The figure shows three views and two pictorial views of one solid part (mm, origin at its lowest corner). Answer the questions. Coordinates: 2 decimals unless noted, no trailing zeros. Loops run counter-clockwise (first coordinate to the right, second up) from the corner with the lowest first, then second, coordinate; pieces in that order, holes last. Notation, with made-up numbers: (-8, 8) -> (5, 8) arc R24 ccw to (5, 23) -> close; hole circle Ø4 at (27.25, 27.25). An arc over 180 degrees is marked (long way). Answer in a Markdown table with one row per item.
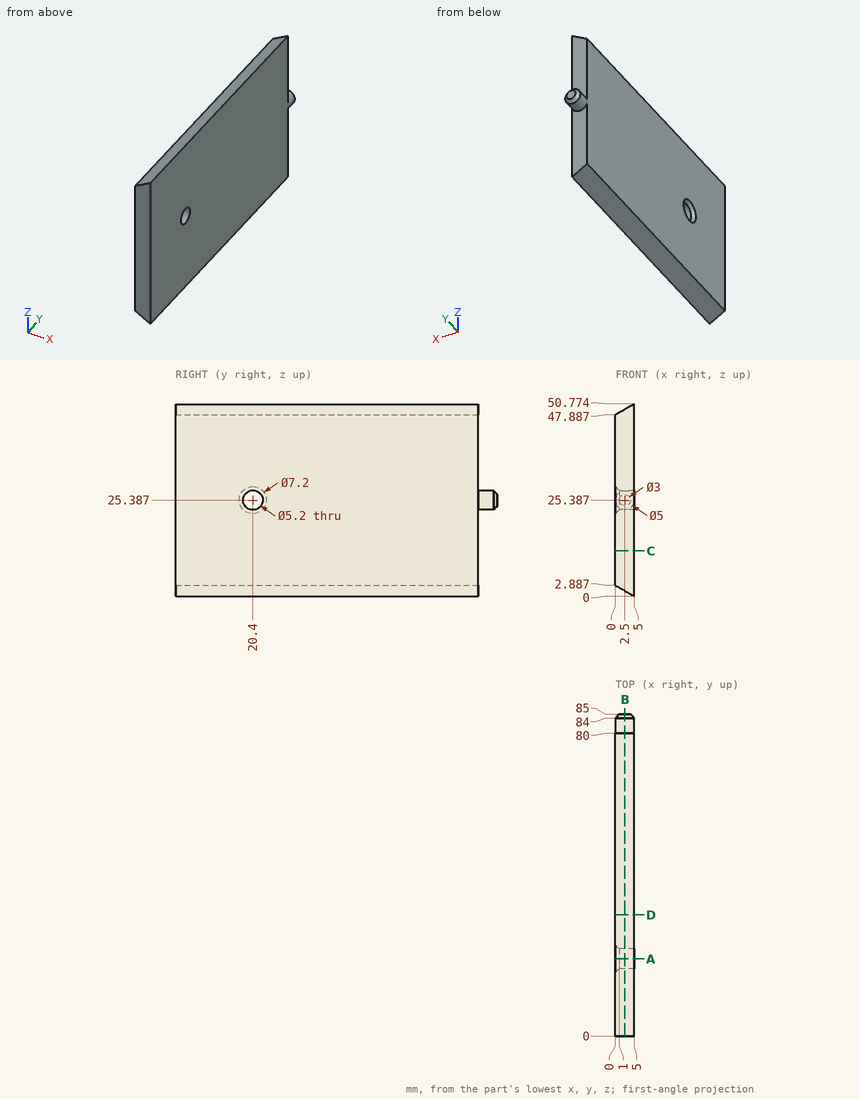
Item 1: A cutting plane is placed at B-B, the plane x = 2.5. Determine the outline of the cut face in (y, z).
Findings below:
| item | result |
|---|---|
| outline | (0, 1.44) -> (80, 1.44) -> (80, 22.89) -> (84, 22.89) -> (85, 23.89) -> (85, 26.89) -> (84, 27.89) -> (80, 27.89) -> (80, 49.33) -> (0, 49.33) -> close; hole circle Ø5.2 at (20.4, 25.39) |
Item 2: A cutting plane is placed at D-D, the plane y = 32. Determine the outline of the cut face in (x, z).
Findings below:
| item | result |
|---|---|
| outline | (0, 2.89) -> (5, 0) -> (5, 50.77) -> (0, 47.89) -> close |
Item 3: Find the intervals of material crossed by probe 1 along Y at (x, z) = (4.75, 39); probe 2 along Y at (x, z) = (0.65, 23) (1 decimal); probe 3 along Z at (x, y) = (4.5, 33) (1 decimal), in increasing order.
Findings below:
| item | result |
|---|---|
| probe 1 | y = 0 to 80 |
| probe 2 | y = 0 to 18.7, 22.1 to 80 |
| probe 3 | z = 0.3 to 50.5 |
Item 4: A cutting plane is placed at C-C, the plane z = 12. Determine the outline of the cut face in (x, y).
Findings below:
| item | result |
|---|---|
| outline | (0, 0) -> (5, 0) -> (5, 80) -> (0, 80) -> close |
Item 5: A cutting plane is placed at A-A, the plane y = 20.4. Determine the outline of the cut face in (x, z).
Findings below:
| item | result |
|---|---|
| outline | (0, 2.89) -> (5, 0) -> (5, 22.79) -> (1, 22.79) -> (0, 21.79) -> close; (0, 28.99) -> (1, 27.99) -> (5, 27.99) -> (5, 50.77) -> (0, 47.89) -> close |
Item 6: A flat-ended cylindrical pin translates along its axis: pin 1 Ø1 at (x, z) = (2.5, 5) entering from +Y. Find the tip coordinate at first contact, or state that the pin passes through.
Findings below:
| item | result |
|---|---|
| pin 1 | stops at y = 80 |
